Design review of the part shown in the three views and the two pictorial views. Dimensions are in mm from the part's minimum x, y and z. A direction names the side the tool comes from. Give positions to 0.01 mm unless a question says otherwise; leave off trailing zeros. Loops run counter-clockwise (first coordinate to the right, second up) from the corner with the lowest first, then second, coordinate; pieces in that order, holes last. Notation, with made-up numbers: M 53,68.25 L 60,68.25 A17 cw 60,74.25 Z; hole C 88,72 d6. An arc over 180 degrees is marked long. Return JSON: item names as keys, results as strings. Group by question number.
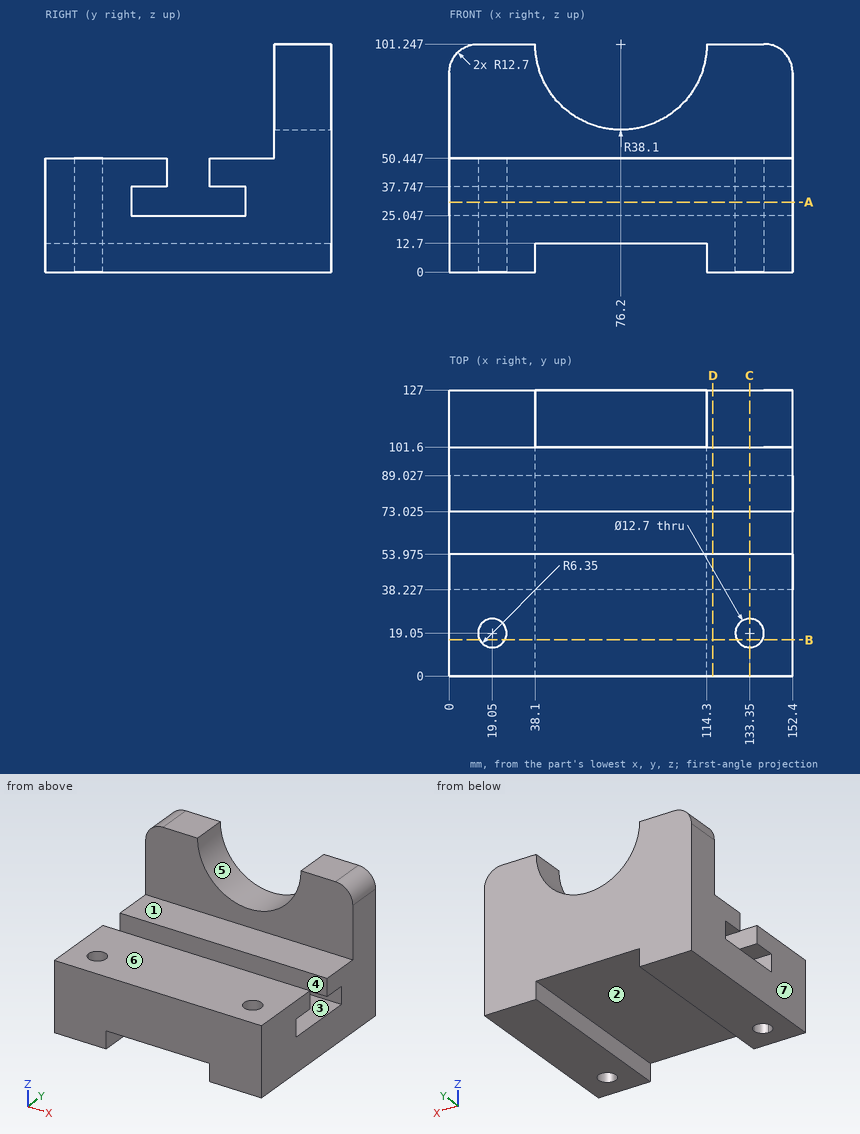
(1) For probe 1 along X at (y, z) = (19, 36); probe 2 along Z at (x, y) = (145, 82); probe 3 along Y at (x, z) = (133.35, 32), list the stretches that pass through material, from the lowest coordinate up.
(2) For the marked faces 1, 2, 3 and 4, list the 3-axis set-ups (+Z, -Z, +X, -X, +Y, -Y) from which the entire face can be reached by the end or side of a thin tool; tool diameter is ignored.
(3) Mouldability with a two-part tool opening along X and no side actions: class the marked faces 5, 6 and 7 as released by +X, released by -X, zero draft, split by the parting line, or undercut.
(4) Add section A-A (z = 31). Write out the cut boundary in (x, y), and give its area (3 significant figures).
(5) Add section C-C (x = 133.35). Write out the cut boundary in (y, z) (1 decimal), and give its area (3 significant figures).
(6) For pin 1 (20.5 mm diameter, centred on x = 133.35, y = 19.05, fed in from +Z); pin 2 (8 mm diameter, centred on x = 60.5, y = 44.5, fed in from -Z), all flat-tipped, find the tip position at first contact; note any pin that passes through.
(7) Add section D-D (x = 117). Write out the cut boundary in (y, z) (1 decimal), and give its area (3 significant figures).
(8) Add section B-B (y = 16). Write out the cut boundary in (x, z), and give its area (3 significant figures).
Verdict:
{
 "1": {"probe 1": "x = 0 to 12.7, 25.4 to 127, 139.7 to 152.4", "probe 2": "z = 0 to 25.05, 37.75 to 50.45", "probe 3": "y = 0 to 12.7, 25.4 to 38.23, 89.03 to 127"},
 "2": {"face 1": "+Z, +X, -X, -Y", "face 2": "-Z, +Y, -Y", "face 3": "+X, -X", "face 4": "+Z, +X, -X"},
 "3": {"face 5": "undercut", "face 6": "zero draft", "face 7": "released by -X"},
 "4": {"outline": "M 0,0 L 152.4,0 L 152.4,38.23 L 0,38.23 Z; M 0,89.03 L 152.4,89.03 L 152.4,127 L 0,127 Z; hole C 19.05,19.05 d12.7; hole C 133.35,19.05 d12.7", "area": "11,400 mm²"},
 "5": {"outline": "M 0,0 L 12.7,0 L 12.7,50.4 L 0,50.4 Z; M 25.4,0 L 127,0 L 127,101.2 L 101.6,101.2 L 101.6,50.4 L 73,50.4 L 73,37.7 L 89,37.7 L 89,25 L 38.2,25 L 38.2,37.7 L 54,37.7 L 54,50.4 L 25.4,50.4 Z", "area": "6,170 mm²"},
 "6": {"pin 1": "stops at z = 50.45", "pin 2": "stops at z = 12.7"},
 "7": {"outline": "M 0,0 L 127,0 L 127,101.2 L 101.6,101.2 L 101.6,50.4 L 73,50.4 L 73,37.7 L 89,37.7 L 89,25 L 38.2,25 L 38.2,37.7 L 54,37.7 L 54,50.4 L 0,50.4 Z", "area": "6,810 mm²"},
 "8": {"outline": "M 0,0 L 13.48,0 L 13.48,50.45 L 0,50.45 Z; M 24.62,0 L 38.1,0 L 38.1,12.7 L 114.3,12.7 L 114.3,0 L 127.78,0 L 127.78,50.45 L 24.62,50.45 Z; M 138.92,0 L 152.4,0 L 152.4,50.45 L 138.92,50.45 Z", "area": "5,600 mm²"}
}
